The listing builds one solid part. Answer for the finished solid, in the listing's coordinates (mm). Face numbers are marked on the shaded views. A direction names the side the tool comes from. Coordinates: 2 decimals unless noted, no trailing zeros. Loops run counter-clockwise (first coordinate to the right, second up) from the corner with the lowest first, then second, coordinate; pieces in that order, holes last. Notation, with made-up numbers: (68, 64) - (110, 64) arc R11 ccw to (110, 69) - close; hole circle Ø2 at (76.5, 24.5). An arc over 180 degrees is marked (long way). Write each question's results on one line, items separated by ' | '. Start each with the question number.
(1) Find section B-B on y = 210.5. Determine the outline of the cut face in (x, z), then the cut area to 3 significant figures.
(2) For the marked faces 1 and 2, determine the directions among +Z, -Z, +X, -X, +Y, -Y from which every point of the face is accessible in a straight line to the end or side of a thin tool.
(3) Given pin 1 Ø4 at (x, y) = (22.86, 16.53) entering from +Z; pin 2 Ø5 at (x, z) = (19.5, 10) entering from +Y; pin 3 Ø4 at (y, z) = (186, 7) entering from -X; pin 4 Ø1 at (x, z) = (-11, 2) entering from -Y, each flat-ended and moving along its own axis, determine where each tip first touches the part or whether it passes through.
(4) Determine the mould class of the marked faces 3 and 4 for opening direction Y: released by +Y, released by -Y, zero draft, split by the parting line, or undercut.
(5) Consider line 1 (Y direction, x = 0, z = 4.25); line 2 (Y direction, x = 0, z = 8.5); line 3 (Y direction, x = 12.5, z = 4.25). Determine where each line is inside the solid, lowest interval first. Write a range as from..to.
(6) Find section A-A on y = 116. Determine the outline of the cut face in (x, z) (1 decimal), then the cut area to 3 significant figures.
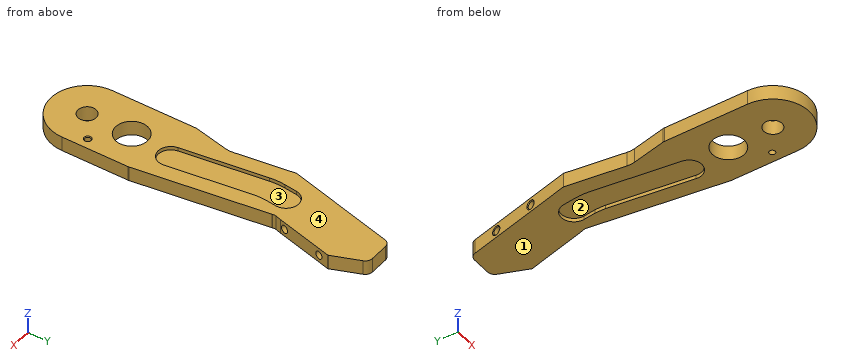
from build123d import *

# Parameters (mm, degrees)
SKETCH1_R                         = 7.9375
SKETCH1_R_2                       = 13.9954
BOSS_EXTRUDE1_DEPTH               = 12.7
FILLET3_R                         = 19.05
FILLET1_R                         = 6.35
F_10_CLEARANCE_HOLE2_D            = 5.1054
F_10_CLEARANCE_HOLE2_CSINK_D      = 6.3754
F_10_CLEARANCE_HOLE2_CSINK_ANGLE  = 90
CUT_EXTRUDE1_DEPTH                = 1
CUT_EXTRUDE1_DEPTH_BACK           = 13.7
FILLET2_R                         = 6.35
CUT_EXTRUDE3_DEPTH                = 1
CUT_EXTRUDE3_DEPTH_BACK           = 13.7
F_1_4_CLEARANCE_HOLE1_D           = 6.7564
F_1_4_CLEARANCE_HOLE1_CSINK_D     = 8.0264
F_1_4_CLEARANCE_HOLE1_CSINK_ANGLE = 90
CUT_EXTRUDE4_DEPTH                = 3.175
CUT_EXTRUDE5_DEPTH                = 3.175


with BuildPart() as part:
    # Sketch1 → Boss-Extrude1 (new body)
    with BuildSketch(Plane.XY):
        with BuildLine():
            Line((-24.200430201, 107.448474159), (-31.75, 73.770562428))
            Line((-31.75, 73.770562428), (-31.75, 0))
            ThreePointArc((-31.75, 0), (0, -31.75), (31.75, 0))
            Line((31.75, 0), (31.75, 116.627004246))
            Line((31.75, 116.627004246), (15.676297005, 175.624413942))
            Line((15.676297005, 175.624413942), (31.947601555, 229.990483385))
            Line((31.947601555, 229.990483385), (19.875208624, 261.32607122))
            Line((19.875208624, 261.32607122), (-5.524791376, 261.32607122))
            Line((-5.524791376, 261.32607122), (-32.716068836, 170.47392878))
            Line((-32.716068836, 170.47392878), (-24.200430201, 107.448474159))
        make_face()
        Circle(SKETCH1_R, mode=Mode.SUBTRACT)
        with Locations((0, 39.116)):
            Circle(SKETCH1_R_2, mode=Mode.SUBTRACT)
    extrude(amount=BOSS_EXTRUDE1_DEPTH)

    # Fillet3
    fillet3_edges = [part.edges().sort_by_distance(p)[0] for p in [
        (-24.200430201, 107.448474159, 6.35),
    ]]
    fillet(fillet3_edges, radius=FILLET3_R)

    # Fillet1
    fillet1_edges = [part.edges().sort_by_distance(p)[0] for p in [
        (-32.716068836, 170.47392878, 6.35),
        (-5.524791376, 261.32607122, 6.35),
        (19.875208624, 261.32607122, 6.35),
        (31.947601555, 229.990483385, 6.35),
        (15.676297005, 175.624413942, 6.35),
        (31.75, 116.627004246, 6.35),
        (-31.75, 73.770562428, 6.35),
    ]]
    fillet(fillet1_edges, radius=FILLET1_R)

    # #10 Clearance Hole2 (through all)
    with Locations(Plane.XY.offset(12.7)):
        with Locations((22.86, 16.52905)):
            CounterSinkHole(F_10_CLEARANCE_HOLE2_D / 2, F_10_CLEARANCE_HOLE2_CSINK_D / 2, counter_sink_angle=F_10_CLEARANCE_HOLE2_CSINK_ANGLE)

    # Sketch17 → Cut-Extrude1 (cut, two sides)
    with BuildSketch(Plane(origin=(0, 0, 0), x_dir=(-1, 0, 0), z_dir=(0, 0, -1))) as cut_extrude1_sk:
        with BuildLine():
            Line((-31.75, 58.539367012), (-16.179878819, 173.776051895))
            Line((-16.179878819, 173.776051895), (-31.526685006, 117.446666412))
            ThreePointArc((-31.526685006, 117.446666412), (-31.693923649, 116.619502039), (-31.75, 115.777465753))
            Line((-31.75, 115.777465753), (-31.75, 58.539367012))
        make_face()
    extrude(amount=CUT_EXTRUDE1_DEPTH, mode=Mode.SUBTRACT)
    extrude(cut_extrude1_sk.sketch, amount=-CUT_EXTRUDE1_DEPTH_BACK, mode=Mode.SUBTRACT)

    # Fillet2
    fillet2_edges = [part.edges().sort_by_distance(p)[0] for p in [
        (31.75, 58.539367012, 6.35),
    ]]
    fillet(fillet2_edges, radius=FILLET2_R)

    # Sketch19 → Cut-Extrude3 (cut, two sides)
    with BuildSketch(Plane(origin=(0, 0, 0), x_dir=(-1, 0, 0), z_dir=(0, 0, -1))) as cut_extrude3_sk:
        with BuildLine():
            Line((-17.620933209, 182.121878639), (-30.825593631, 232.902812203))
            Line((-30.825593631, 232.902812203), (-31.167525601, 232.015279853))
            ThreePointArc((-31.167525601, 232.015279853), (-31.587367542, 229.976620184), (-31.325446349, 227.911723628))
            Line((-31.325446349, 227.911723628), (-17.620933209, 182.121878639))
        make_face()
        with BuildLine():
            Line((32.32313572, 171.786806246), (6.880371133, 256.796775922))
            Line((6.880371133, 256.796775922), (31.557248698, 161.897335866))
            Line((31.557248698, 161.897335866), (32.532573251, 169.115851816))
            ThreePointArc((32.532573251, 169.115851816), (32.570321666, 170.462500309), (32.32313572, 171.786806246))
        make_face()
    extrude(amount=CUT_EXTRUDE3_DEPTH, mode=Mode.SUBTRACT)
    extrude(cut_extrude3_sk.sketch, amount=-CUT_EXTRUDE3_DEPTH_BACK, mode=Mode.SUBTRACT)

    # 1/4 Clearance Hole1 (through all)
    with Locations(Plane(origin=(-68.990792956, 17.939803964, 0), x_dir=(0, 0, 1), z_dir=(-0.967814998, 0.251662731, 0))):
        with Locations((6.35, 185.089358388), (6.35, 223.189358388)):
            CounterSinkHole(F_1_4_CLEARANCE_HOLE1_D / 2, F_1_4_CLEARANCE_HOLE1_CSINK_D / 2, counter_sink_angle=F_1_4_CLEARANCE_HOLE1_CSINK_ANGLE)

    # Sketch22 → Cut-Extrude4 (cut)
    with BuildSketch(Plane(origin=(0, 0, 0), x_dir=(-1, 0, 0), z_dir=(0, 0, -1))):
        with BuildLine():
            Line((-5.721549742, 151.036596427), (-15.563924684, 78.191777395))
            ThreePointArc((-15.563924684, 78.191777395), (-6.101580096, 65.772977875), (6.317219423, 75.235322463))
            Line((6.317219423, 75.235322463), (16.227356213, 148.58165658))
            ThreePointArc((16.227356213, 148.58165658), (16.127581623, 152.147558265), (14.895920611, 155.495486123))
            ThreePointArc((14.895920611, 155.495486123), (5.286667697, 150.045412833), (-4.233623122, 155.649438455))
            ThreePointArc((-4.233623122, 155.649438455), (-5.148189302, 153.664409279), (-5.653787894, 151.538111511))
            Line((-5.653787894, 151.538111511), (-5.721549742, 151.036596427))
        make_face()
        with BuildLine():
            ThreePointArc((14.895920611, 155.495486123), (5.375629793, 161.099511745), (-4.233623122, 155.649438455))
            ThreePointArc((-4.233623122, 155.649438455), (5.286667697, 150.045412833), (14.895920611, 155.495486123))
        make_face()
        with BuildLine():
            Line((-6.858366152, 170.484855738), (-5.647114594, 160.285630757))
            Line((-5.647114594, 160.285630757), (-5.587433271, 159.783090025))
            ThreePointArc((-5.587433271, 159.783090025), (-5.116122344, 157.648930204), (-4.233623122, 155.649438455))
            ThreePointArc((-4.233623122, 155.649438455), (5.375629793, 161.099511745), (14.895920611, 155.495486123))
            ThreePointArc((14.895920611, 155.495486123), (16.181306062, 158.823157086), (16.338459931, 162.386991041))
            Line((16.338459931, 162.386991041), (15.06752705, 173.088756754))
            ThreePointArc((15.06752705, 173.088756754), (2.802629941, 182.749752847), (-6.858366152, 170.484855738))
        make_face()
        with BuildLine():
            ThreePointArc((14.895920611, 155.495486123), (16.127581623, 152.147558265), (16.227356213, 148.58165658))
            ThreePointArc((16.227356213, 148.58165658), (16.719229878, 155.480812344), (16.338459931, 162.386991041))
            ThreePointArc((16.338459931, 162.386991041), (16.181306062, 158.823157086), (14.895920611, 155.495486123))
        make_face()
        with BuildLine():
            ThreePointArc((-5.647114594, 160.285630757), (-5.608314081, 155.660501807), (-5.721549742, 151.036596427))
            Line((-5.721549742, 151.036596427), (-5.653787894, 151.538111511))
            ThreePointArc((-5.653787894, 151.538111511), (-5.148189302, 153.664409279), (-4.233623122, 155.649438455))
            ThreePointArc((-4.233623122, 155.649438455), (-5.116122344, 157.648930204), (-5.587433271, 159.783090025))
            Line((-5.587433271, 159.783090025), (-5.647114594, 160.285630757))
        make_face()
    extrude(amount=-CUT_EXTRUDE4_DEPTH, mode=Mode.SUBTRACT)

    # Sketch23 → Cut-Extrude5 (cut)
    with BuildSketch(Plane.XY.offset(12.7)):
        with BuildLine():
            ThreePointArc((-6.317219423, 75.235322463), (6.101580096, 65.772977875), (15.563924684, 78.191777395))
            Line((15.563924684, 78.191777395), (5.721549742, 151.036596427))
            Line((5.721549742, 151.036596427), (5.653787894, 151.538111511))
            ThreePointArc((5.653787894, 151.538111511), (5.148189302, 153.664409279), (4.233623122, 155.649438455))
            ThreePointArc((4.233623122, 155.649438455), (-5.286667697, 150.045412833), (-14.895920611, 155.495486123))
            ThreePointArc((-14.895920611, 155.495486123), (-16.127581623, 152.147558265), (-16.227356213, 148.58165658))
            Line((-16.227356213, 148.58165658), (-6.317219423, 75.235322463))
        make_face()
        with BuildLine():
            ThreePointArc((-14.895920611, 155.495486123), (-5.286667697, 150.045412833), (4.233623122, 155.649438455))
            ThreePointArc((4.233623122, 155.649438455), (-5.375629793, 161.099511745), (-14.895920611, 155.495486123))
        make_face()
        with BuildLine():
            Line((5.587433271, 159.783090025), (5.647114594, 160.285630757))
            Line((5.647114594, 160.285630757), (6.858366152, 170.484855738))
            ThreePointArc((6.858366152, 170.484855738), (-2.802629941, 182.749752847), (-15.06752705, 173.088756754))
            Line((-15.06752705, 173.088756754), (-16.338459931, 162.386991041))
            ThreePointArc((-16.338459931, 162.386991041), (-16.181306062, 158.823157086), (-14.895920611, 155.495486123))
            ThreePointArc((-14.895920611, 155.495486123), (-5.375629793, 161.099511745), (4.233623122, 155.649438455))
            ThreePointArc((4.233623122, 155.649438455), (5.116122344, 157.648930204), (5.587433271, 159.783090025))
        make_face()
        with BuildLine():
            ThreePointArc((-16.338459931, 162.386991041), (-16.719229878, 155.480812344), (-16.227356213, 148.58165658))
            ThreePointArc((-16.227356213, 148.58165658), (-16.127581623, 152.147558265), (-14.895920611, 155.495486123))
            ThreePointArc((-14.895920611, 155.495486123), (-16.181306062, 158.823157086), (-16.338459931, 162.386991041))
        make_face()
        with BuildLine():
            Line((5.653787894, 151.538111511), (5.721549742, 151.036596427))
            ThreePointArc((5.721549742, 151.036596427), (5.608314081, 155.660501807), (5.647114594, 160.285630757))
            Line((5.647114594, 160.285630757), (5.587433271, 159.783090025))
            ThreePointArc((5.587433271, 159.783090025), (5.116122344, 157.648930204), (4.233623122, 155.649438455))
            ThreePointArc((4.233623122, 155.649438455), (5.148189302, 153.664409279), (5.653787894, 151.538111511))
        make_face()
    extrude(amount=-CUT_EXTRUDE5_DEPTH, mode=Mode.SUBTRACT)


solid = part.part
Values:
1) outline: (-18.92, 0) - (25, 0) - (25, 12.7) - (-18.92, 12.7) - close | area: 558 mm²
2) face 1: -Z, +X, -X, +Y, -Y | face 2: -Z
3) pin 1: passes through | pin 2: stops at y = 261.15 | pin 3: stops at x = -25.81 | pin 4: stops at y = -29.96
4) face 3: undercut | face 4: zero draft
5) line 1: y = -31.75..-7.94, 7.94..25.12, 53.11..188.51, 193.98..227.88, 233.35..261.33 | line 2: y = -31.75..-7.94, 7.94..25.12, 53.11..188.55, 193.94..227.92, 233.3..261.33 | line 3: y = -29.19..32.82, 45.41..185.26, 190.73..224.63, 230.1..261.33
6) outline: (-25.4, 0) - (-11.8, 0) - (-11.8, 3.2) - (10.5, 3.2) - (10.5, 0) - (24, 0) - (24, 12.7) - (10.5, 12.7) - (10.5, 9.5) - (-11.8, 9.5) - (-11.8, 12.7) - (-25.4, 12.7) - close | area: 485 mm²
